Build history of the part. All positions in model axes, mm. Face numbers are marked on the shaded views. A direction names the side the tool comes from. Give positions to 0.01 mm unless a question says otherwise; leave off trailing zeros. Write each loop counter-clockwise with the first axis right and the second up, starting at its lowest first coordinate (ties: lowest second). Pieces come first, ordered by that corner, then holes. Notation, with made-up numbers: (36, 68.25) -> (87, 68.25) arc R14 cw to (87, 79.25) -> close; hole circle Ø5 at (-2, 66.25). An arc over 180 degrees is marked (long way). Write item = value, one per line. Start each with the question number.
Q1. Tool access for the marked faces 1 and 2: list every direction of +Z, -Z, +X, -X, +Y, -Y with a clear straight run to the whole face (end or side of a thin tool).
Q2. Saw through at C-C, the plane x = 19.55. List the corners of the cut face in (y, z), then the cut area to 3 significant figures.
Q3. Saw through at D-D, the plane y = 12.5. List the corners of the cut face in (x, z).
Q4. Wall check: line 1 (X direction, y = 0.4, z = -9.05); line 2 (Z direction, x = 3.55, y = 0.4); line 3 (Y direction, x = 6, z = -19.5). Give the ranges that are in metal, low to high.
Q5. Saw through at A-A, the plane z = -25. List the corners of the cut face in (x, y), then the cut area to 3 significant figures.
Q6. Drop flat-ended pins along their axis: P1, Ø3, axis at x = 24.5, y = 15, coming from the -Z side; P2, Ø1.9, axis at x = 35.55, z = -9.05, coming from the -Y side; P3, Ø1, axis at y = 8.5, z = -24.5, coming from the -X side; P4, Ø5, axis at x = 31.5, y = 5.5, coming from the +Z side. Give the stop position or say it passes through.
Q7. Saw through at B-B, the plane x = 3. List the corners of the cut face in (y, z), then the cut area to 3 significant figures.
from build123d import *

# Parameters (mm, degrees)
SKETCH1_W           = 39.1
SKETCH1_H           = 44.6
BOSS_EXTRUDE1_DEPTH = 1.5
SKETCH2_R           = 1.6
CUT_EXTRUDE1_DEPTH  = 1.5
SKETCH3_R           = 16
BOSS_EXTRUDE2_DEPTH = 16.5
FILLET1_R           = 2


with BuildPart() as part:
    # Sketch1 → Boss-Extrude1 (new body)
    with BuildSketch(Plane(origin=(0, 0, 0), x_dir=(1, 0, 0), z_dir=(0, 1, 0))):
        with Locations((19.55, 22.3)):
            Rectangle(SKETCH1_W, SKETCH1_H)
    extrude(amount=BOSS_EXTRUDE1_DEPTH)

    # Sketch2 → Cut-Extrude1 (cut)
    with BuildSketch(Plane(origin=(0, 1.5, 0), x_dir=(1, 0, 0), z_dir=(0, 1, 0))):
        with Locations((35.55, 9.05)):
            Circle(SKETCH2_R)
        with Locations((35.55, 41.05)):
            Circle(SKETCH2_R)
        with Locations((3.55, 41.05)):
            Circle(SKETCH2_R)
        with Locations((3.55, 9.05)):
            Circle(SKETCH2_R)
    extrude(amount=-CUT_EXTRUDE1_DEPTH, mode=Mode.SUBTRACT)

    # Sketch3 → Boss-Extrude2 (add)
    with BuildSketch(Plane(origin=(0, 1.5, 0), x_dir=(1, 0, 0), z_dir=(0, 1, 0))):
        with Locations((19.55, 25)):
            Circle(SKETCH3_R)
    extrude(amount=BOSS_EXTRUDE2_DEPTH)

    # Fillet1
    fillet1_edges = [part.edges().sort_by_distance(p)[0] for p in [
        (3.55, 18, -25),
    ]]
    fillet(fillet1_edges, radius=FILLET1_R)


solid = part.part
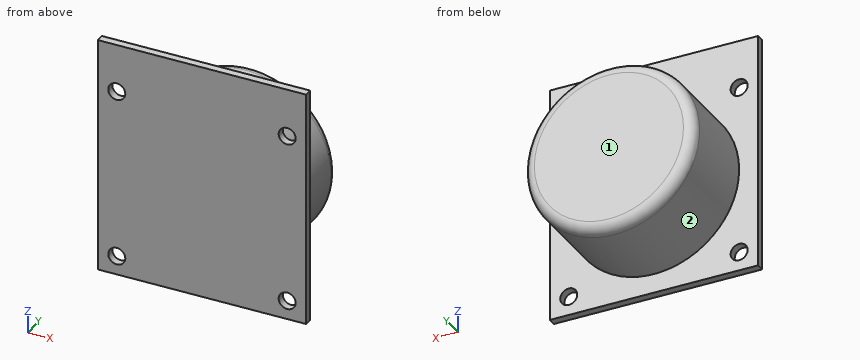
Report:
q1.face_1 = +Z, -Z, +X, -X, +Y
q1.face_2 = +Y
q2.outline = (0, -44.6) -> (1.5, -44.6) -> (1.5, -41) -> (16, -41) arc R2 ccw to (18, -39) -> (18, -11) arc R2 ccw to (16, -9) -> (1.5, -9) -> (1.5, 0) -> (0, 0) -> close
q2.area = 593 mm2
q3.outline = circle Ø32 at (19.55, -25)
q4.line_1 = 0 to 1.95, 5.15 to 33.95, 37.15 to 39.1
q4.line_2 = -44.6 to -42.65, -39.45 to -10.65, -7.45 to 0
q4.line_3 = 0 to 17.9
q5.outline = (0, 0) -> (39.1, 0) -> (39.1, 1.5) -> (35.55, 1.5) -> (35.55, 16) arc R2 ccw to (33.55, 18) -> (5.55, 18) arc R2 ccw to (3.55, 16) -> (3.55, 1.5) -> (0, 1.5) -> close
q5.area = 585 mm2
q6.P1 = -40.62
q6.P2 = through
q6.P3 = 3.55
q6.P4 = -12.09
q7.outline = (0, -44.6) -> (1.5, -44.6) -> (1.5, -42.55) -> (0, -42.55) -> close; (0, -39.55) -> (1.5, -39.55) -> (1.5, -10.55) -> (0, -10.55) -> close; (0, -7.55) -> (1.5, -7.55) -> (1.5, 0) -> (0, 0) -> close
q7.area = 57.9 mm2
